```python
from build123d import *

# Parameters (mm, degrees)
F0_R         = 38.1
F0_R_2       = 2.54
F0_R_3       = 5.08
F1_DEPTH     = 5.08
F5_T1_DEPTH  = 14.1990316571
F5_T6_ANGLE  = 276.3793702084
F5_T8_ANGLE  = 131.8103148958
F5_T10_ANGLE = 180
F5_T12_ANGLE = 131.8103148958
F5_T20_ANGLE = 276.3793702084
F5_T22_ANGLE = 131.8103148958
F5_T24_ANGLE = 180
F5_T26_ANGLE = 131.8103148958
F5_T32_ANGLE = 270
F5_T34_ANGLE = 90
F5_T36_ANGLE = 90
F5_T38_ANGLE = 270


# Not quite as in the source:
# - a fillet or chamfer that OpenCascade refuses, or shapes differently, is made with other operations: its cross-section is extruded or revolved along the edge and cut away or added


with BuildPart() as f1:
    # F0 (on Front) → F1 (new body)
    with BuildSketch(Plane.XZ):
        Circle(F0_R)
        with BuildLine():
            ThreePointArc((16.9333333333, 18.9320422095), (0, -25.4), (-16.9333333333, 18.9320422095))
            ThreePointArc((-16.9333333333, 18.9320422095), (-10.1076233556, 19.9957620574), (-6.35, 14.1990316571))
            Line((-6.35, 14.1990316571), (-6.35, 0))
            ThreePointArc((-6.35, 0), (-4.4901280605, -4.4901280605), (0, -6.35))
            ThreePointArc((0, -6.35), (4.4901280605, -4.4901280605), (6.35, 0))
            Line((6.35, 0), (6.35, 14.1990316571))
            ThreePointArc((6.35, 14.1990316571), (10.1076233556, 19.9957620574), (16.9333333333, 18.9320422095))
        make_face(mode=Mode.SUBTRACT)
        Circle(F0_R_2, mode=Mode.SUBTRACT)
        with Locations((0, 25.4)):
            Circle(F0_R_3, mode=Mode.SUBTRACT)
    extrude(amount=F1_DEPTH)


with BuildPart() as f3:
    # F2 (on Right) → F3 (revolve)
    with BuildSketch(Plane.YZ):
        with BuildLine():
            ThreePointArc((-3.54, 38.1), (-2.54, 37.1), (-1.54, 38.1))
            Line((-1.54, 38.1), (-3.54, 38.1))
        make_face()
        with BuildLine():
            Line((-3.54, 38.1), (-1.54, 38.1))
            ThreePointArc((-1.54, 38.1), (-2.54, 39.1), (-3.54, 38.1))
        make_face()
    revolve(axis=Axis((0, 0, 0), (0, -1, 0)))


with BuildPart() as f1_1:
    add(f1.part)

    # F4: cut F3
    add(f3.part, mode=Mode.SUBTRACT)

    # F5: chamfer of 0.508 on 22 edges, made by hand

    # F5_s2 → F5_t1 (cut)
    with BuildSketch(Plane.XY):
        Polygon((-6.35, -4.572), (-5.842, -5.08), (-6.35, -5.08), align=None)
        Polygon((6.35, -4.572), (5.842, -5.08), (6.35, -5.08), align=None)
        Polygon((-5.842, 0), (-6.35, -0.508), (-6.35, 0), align=None)
        Polygon((5.842, 0), (6.35, -0.508), (6.35, 0), align=None)
    extrude(amount=F5_T1_DEPTH, mode=Mode.SUBTRACT)

    # F5_s3 → F5_t4 (revolve, cut)
    with BuildSketch(Plane.XY):
        Polygon((38.1, -4.572), (37.592, -5.08), (38.1, -5.08), align=None)
    revolve(axis=Axis((0, -5.08, 0), (0, -1, 0)), mode=Mode.SUBTRACT)

    # F5_s5 → F5_t6 (revolve, cut)
    with BuildSketch(Plane(origin=(0, 0, 0), x_dir=(0, 1, 0), z_dir=(-0.7453559925, 0, 0.6666666667))):
        Polygon((-4.572, -25.4), (-5.08, -25.908), (-5.08, -25.4), align=None)
    revolve(axis=Axis((0, -5.08, 0), (0, 1, 0)), revolution_arc=F5_T6_ANGLE, mode=Mode.SUBTRACT)

    # F5_s7 → F5_t8 (revolve, cut)
    with BuildSketch(Plane(origin=(0, 0, 0), x_dir=(0, 1, 0), z_dir=(-0.7453559925, 0, -0.6666666667))):
        Polygon((-4.572, -25.4), (-5.08, -25.908), (-5.08, -25.4), align=None)
    revolve(axis=Axis((-12.7, -5.08, 14.1990316571), (0, 1, 0)), revolution_arc=F5_T8_ANGLE, mode=Mode.SUBTRACT)

    # F5_s9 → F5_t10 (revolve, cut)
    with BuildSketch(Plane.XY):
        Polygon((6.35, -4.572), (5.842, -5.08), (6.35, -5.08), align=None)
    revolve(axis=Axis((0, -5.08, 0), (0, 1, 0)), revolution_arc=F5_T10_ANGLE, mode=Mode.SUBTRACT)

    # F5_s11 → F5_t12 (revolve, cut)
    with BuildSketch(Plane.XY.offset(14.1990316571)):
        Polygon((6.35, -4.572), (5.842, -5.08), (6.35, -5.08), align=None)
    revolve(axis=Axis((12.7, -5.08, 14.1990316571), (0, 1, 0)), revolution_arc=F5_T12_ANGLE, mode=Mode.SUBTRACT)

    # F5_s13 → F5_t14 (revolve, cut)
    with BuildSketch(Plane.XY):
        Polygon((2.54, -4.572), (3.048, -5.08), (2.54, -5.08), align=None)
    revolve(axis=Axis((0, -5.08, 0), (0, -1, 0)), mode=Mode.SUBTRACT)

    # F5_s15 → F5_t16 (revolve, cut)
    with BuildSketch(Plane.XY.offset(25.4)):
        Polygon((5.08, -4.572), (5.588, -5.08), (5.08, -5.08), align=None)
    revolve(axis=Axis((0, -5.08, 25.4), (0, -1, 0)), mode=Mode.SUBTRACT)

    # F5_s17 → F5_t18 (revolve, cut)
    with BuildSketch(Plane.XY):
        Polygon((38.1, -0.508), (37.592, 0), (38.1, 0), align=None)
    revolve(axis=Axis((0, 0, 0), (0, -1, 0)), mode=Mode.SUBTRACT)

    # F5_s19 → F5_t20 (revolve, cut)
    with BuildSketch(Plane(origin=(0, 0, 0), x_dir=(0, 1, 0), z_dir=(-0.7453559925, 0, 0.6666666667))):
        Polygon((0, -25.908), (-0.508, -25.4), (0, -25.4), align=None)
    revolve(axis=Axis((0, 0, 0), (0, 1, 0)), revolution_arc=F5_T20_ANGLE, mode=Mode.SUBTRACT)

    # F5_s21 → F5_t22 (revolve, cut)
    with BuildSketch(Plane(origin=(0, 0, 0), x_dir=(0, 1, 0), z_dir=(-0.7453559925, 0, -0.6666666667))):
        Polygon((0, -25.908), (-0.508, -25.4), (0, -25.4), align=None)
    revolve(axis=Axis((-12.7, 0, 14.1990316571), (0, 1, 0)), revolution_arc=F5_T22_ANGLE, mode=Mode.SUBTRACT)

    # F5_s23 → F5_t24 (revolve, cut)
    with BuildSketch(Plane.XY):
        Polygon((-5.842, 0), (-6.35, -0.508), (-6.35, 0), align=None)
    revolve(axis=Axis((0, 0, 0), (0, -1, 0)), revolution_arc=F5_T24_ANGLE, mode=Mode.SUBTRACT)

    # F5_s25 → F5_t26 (revolve, cut)
    with BuildSketch(Plane.XY.offset(14.1990316571)):
        Polygon((5.842, 0), (6.35, -0.508), (6.35, 0), align=None)
    revolve(axis=Axis((12.7, 0, 14.1990316571), (0, 1, 0)), revolution_arc=F5_T26_ANGLE, mode=Mode.SUBTRACT)

    # F5_s27 → F5_t28 (revolve, cut)
    with BuildSketch(Plane.XY):
        Polygon((3.048, 0), (2.54, -0.508), (2.54, 0), align=None)
    revolve(axis=Axis((0, 0, 0), (0, -1, 0)), mode=Mode.SUBTRACT)

    # F5_s29 → F5_t30 (revolve, cut)
    with BuildSketch(Plane.XY.offset(25.4)):
        Polygon((5.588, 0), (5.08, -0.508), (5.08, 0), align=None)
    revolve(axis=Axis((0, 0, 25.4), (0, -1, 0)), mode=Mode.SUBTRACT)

    # F5_s31 → F5_t32 (revolve, cut)
    with BuildSketch(Plane.YZ):
        with BuildLine():
            Line((-1.1201408521, 38.1), (-1.5984488409, 37.7631299735))
            ThreePointArc((-1.5984488409, 37.7631299735), (-1.5560027564, 37.921816318), (-1.54, 38.1))
            Line((-1.54, 38.1), (-1.1201408521, 38.1))
        make_face()
    revolve(axis=Axis((0, -1.54, 0), (0, -1, 0)), revolution_arc=F5_T32_ANGLE, mode=Mode.SUBTRACT)

    # F5_s33 → F5_t34 (revolve, cut)
    with BuildSketch(Plane.XY):
        with BuildLine():
            Line((38.1, -1.1201408521), (37.7631299735, -1.5984488409))
            ThreePointArc((37.7631299735, -1.5984488409), (37.921816318, -1.5560027564), (38.1, -1.54))
            Line((38.1, -1.54), (38.1, -1.1201408521))
        make_face()
    revolve(axis=Axis((0, -1.54, 0), (0, -1, 0)), revolution_arc=F5_T34_ANGLE, mode=Mode.SUBTRACT)

    # F5_s35 → F5_t36 (revolve, cut)
    with BuildSketch(Plane.XY):
        with BuildLine():
            Line((37.7631299735, -3.4815511591), (38.1, -3.9598591479))
            Line((38.1, -3.9598591479), (38.1, -3.54))
            ThreePointArc((38.1, -3.54), (37.921816318, -3.5239972436), (37.7631299735, -3.4815511591))
        make_face()
    revolve(axis=Axis((0, -3.54, 0), (0, -1, 0)), revolution_arc=F5_T36_ANGLE, mode=Mode.SUBTRACT)

    # F5_s37 → F5_t38 (revolve, cut)
    with BuildSketch(Plane.YZ):
        with BuildLine():
            Line((-3.4815511591, 37.7631299735), (-3.9598591479, 38.1))
            Line((-3.9598591479, 38.1), (-3.54, 38.1))
            ThreePointArc((-3.54, 38.1), (-3.5239972436, 37.921816318), (-3.4815511591, 37.7631299735))
        make_face()
    revolve(axis=Axis((0, -3.54, 0), (0, -1, 0)), revolution_arc=F5_T38_ANGLE, mode=Mode.SUBTRACT)


solid = f1_1.part
```
Verification items for the finished model (mm, model axes). A direction names the side the tool comes from. Coordinates: 2 decimals unless noted, no trailing zeros. Order: outer loops, then holes, each group sorted by start corner. A loop starts at its lowest first (then second) coordinate and runs counter-clockwise, first axis right, second up. Notation, with made-up numbers: (6, 79) - (24, 79) arc R24 cw to (24, 112) - close; hole circle Ø8 at (34.5, 48). An arc over 180 degrees is marked (long way). Return JSON: item names as keys, results as strings.
(1) Mould release check, pull along X, two halves, no side actions. Record for faces 4 (the cylindrical face through (-30.235, -0.81, -23.183)), 5 (the flat face through (-1, -5.08, 9)), 6 (the cylindrical face through (-0.661, -2.512, 30.437)): pulls with the +X half, pulls with the -X half, needs draft (parallel to the pull), parting line crosses it, or undercut.
Filled sheet:
{"face 4": "parting line crosses it", "face 5": "needs draft", "face 6": "undercut"}
(2) Access from +Z, -Z, +X, -X, +Y, -Y to the whole of each face (thin tool, end or side, straight path). Record for faces 1 (the conical face through (-0.132, -0.145, -5.985)), 2 (the conical face through (0.13, -4.94, -5.98)), 3 (the flat face through (6.35, -3, 7)).
Filled sheet:
{"face 1": "+Y", "face 2": "-Y", "face 3": "+Y, -Y"}
(3) Thickness scan on line 1 along Z through (x, y) = (0, -3.5); line 2 along Z through (x, y) = (0, -2); line 3 along X through (y, z) = (-3.3, 3.5). Record the ranges inside material, lowest first.
Filled sheet:
{"line 1": "z = -37.78 to -25.4, -6.35 to -2.54, 2.54 to 20.32, 30.48 to 37.78", "line 2": "z = -37.26 to -25.4, -6.35 to -2.54, 2.54 to 20.32, 30.48 to 37.26", "line 3": "x = -37.29 to -25.16, -6.35 to 6.35, 25.16 to 37.29"}
(4) Section check A-A, the plane y = -2.55. Record the cut outline in (x, z), and give its area (3 significant figures).
Filled sheet:
{"outline": "circle Ø74.2 at (0, 0); hole (-16.93, 18.93) arc R25.4 ccw (long way) to (16.93, 18.93) arc R6.35 ccw to (6.35, 14.2) - (6.35, 0) arc R6.35 cw to (-6.35, 0) - (-6.35, 14.2) arc R6.35 ccw to start; hole circle Ø10.16 at (0, 25.4); hole circle Ø5.08 at (0, 0)", "area": "2,640 mm^2"}
(5) Go/stop test with flat-tipped pins: pin 1 (16.5 mm diameter, centred on x = 0, z = 25.4, fed in from -Y); pin 2 (8 mm diameter, centred on x = 17, z = 10, fed in from -Y); pin 3 (2 mm diameter, centred on y = -3, z = -11, fed in from -X); pin 4 (3 mm diameter, centred on y = -1, z = 18, fed in from +X). Record where each tip stops, or that it passes through.
Filled sheet:
{"pin 1": "stops at y = -5.08", "pin 2": "passes through", "pin 3": "stops at x = -36.56", "pin 4": "stops at x = 34.34"}
